Geometry: final body of the model. Coordinates: model frame, mm. A direction names the side the tool comes from. Coordinates: 2 decimals unless noted, no trailing zeros. Loops run counter-clockwise (first coordinate to the right, second up) from the corner with the lowest first, then second, coordinate; pieces in that order, holes last. Notation, with made-up numbers: M 60,-12 L 72,-12 A12 ccw 72,1 Z; hole C 80,78.5 d4. An arc over 180 degrees is marked long. Write item = value, one per line. Start each with the question number.
```python
from build123d import *

# Parameters (mm, degrees)
SKETCH1_W            = 25
SKETCH1_H            = 9.6
BOSS_EXTRUDE1_DEPTH  = 2
SKETCH3_R            = 2.3
CUT_EXTRUDE1_DEPTH   = 14.538463724
SKETCH4_W            = 20.2
SKETCH4_H            = 6.2
CUT_EXTRUDE2_DEPTH   = 0.27
SKETCH5_W            = 40
SKETCH5_H            = 20
BOSS_EXTRUDE2_DEPTH  = 4
M3_CLEARANCE_HOLE1_D = 3.2
SKETCH9_W            = 40
SKETCH9_H            = 2
BOSS_EXTRUDE4_DEPTH  = 20
BOSS_EXTRUDE5_DEPTH  = 1.5
FILLET1_R            = 2
FILLET1_OF_MIRROR1_R = 2
M3_CLEARANCE_HOLE2_D = 3.2


with BuildPart() as part:
    # Sketch1 → Boss-Extrude1 (new body)
    with BuildSketch(Plane(origin=(0, 0, 0), x_dir=(1, 0, 0), z_dir=(0, 1, 0))):
        Rectangle(SKETCH1_W, SKETCH1_H)
    extrude(amount=BOSS_EXTRUDE1_DEPTH)

    # Sketch3 → Cut-Extrude1 (cut, through all)
    with BuildSketch(Plane(origin=(0, 2, 0), x_dir=(1, 0, 0), z_dir=(0, 1, 0))):
        with Locations(Location((-7, 0, 0), (0, 0, 270))):
            Circle(SKETCH3_R)
        with Locations(Location((7, 0, 0), (0, 0, 270))):
            Circle(SKETCH3_R)
    extrude(amount=-CUT_EXTRUDE1_DEPTH, mode=Mode.SUBTRACT)

    # Sketch4 → Cut-Extrude2 (cut)
    with BuildSketch(Plane(origin=(0, 0, 0), x_dir=(1, 0, 0), z_dir=(0, 1, 0))):
        Rectangle(SKETCH4_W, SKETCH4_H)
    extrude(amount=CUT_EXTRUDE2_DEPTH, mode=Mode.SUBTRACT)

    # Sketch5 → Boss-Extrude2 (add)
    with BuildSketch(Plane(origin=(0, 2, 0), x_dir=(1, 0, 0), z_dir=(0, 1, 0))):
        Rectangle(SKETCH5_W, SKETCH5_H)
    extrude(amount=BOSS_EXTRUDE2_DEPTH)

    # M3 Clearance Hole1 (through all)
    with Locations(Plane(origin=(0, 2, 0), x_dir=(-1, 0, 0), z_dir=(0, -1, 0))):
        with Locations((-7, 0), (7, 0)):
            Hole(M3_CLEARANCE_HOLE1_D / 2)

    # Sketch9 → Boss-Extrude4 (add)
    with BuildSketch(Plane(origin=(0, 6, 0), x_dir=(1, 0, 0), z_dir=(0, 1, 0))):
        with Locations((0, 9)):
            Rectangle(SKETCH9_W, SKETCH9_H)
        with Locations((0, -9)):
            Rectangle(SKETCH9_W, SKETCH9_H)
    extrude(amount=BOSS_EXTRUDE4_DEPTH)

    # Sketch10 → Boss-Extrude5 (add)
    with BuildSketch(Plane.ZY.offset(12.5)):
        Polygon((-8, 6), (-8, 26), (0, 6), align=None)
        Polygon((8, 6), (0, 6), (8, 26), align=None)
    boss_extrude5 = extrude(amount=BOSS_EXTRUDE5_DEPTH)

    # Fillet1
    fillet1_edges = [part.edges().sort_by_distance(p)[0] for p in [
        (-13.25, 6, 0),
    ]]
    fillet(fillet1_edges, radius=FILLET1_R)

    # Mirror1: Boss-Extrude5 across plane
    add(boss_extrude5.mirror(Plane.ZY))

    # Fillet1 of Mirror1
    fillet1_of_mirror1_edges = [part.edges().sort_by_distance(p)[0] for p in [
        (13.25, 6, 0),
    ]]
    fillet(fillet1_of_mirror1_edges, radius=FILLET1_OF_MIRROR1_R)

    # M3 Clearance Hole2 (through all)
    with Locations(Plane.XY.offset(10)):
        with Locations((-17.5, 21), (17.5, 21), (17.5, 11), (-17.5, 11), (0, 21), (0, 11)):
            Hole(M3_CLEARANCE_HOLE2_D / 2)


solid = part.part
```
Item 1: Section query A-A (x = 17.5). Return the cut outline in (y, z).
Item 2: Pull-direction query (Y, two-part tool) for faces 1 (the cylindrical face through (-6.309, 1.147, 2.194)), 2 (the cylindrical face through (0.208, 22.586, -9.014)), 3 (the cylindrical face through (0.35, 9.44, -9.01)), 4 (the flat face through (0, 26, 9)); classes: released by +Y, released by -Y, zero draft, split by the parting line, or undercut.
Item 3: First-contact query: pin 1 (3 mm diameter, centred on x = -5, z = 0.5, fed in from -Y); pin 2 (1.9 mm diameter, centred on x = -17.5, y = 21, fed in from -Z) (1 decimal); pin 3 (3 mm diameter, centred on x = 18, z = -1.5, fed in from +Y); pin 4 (3.5 mm diameter, centred on x = 7, z = 0, fed in from -Y). Flat tips, straight axial feed; report the tip coordinate or a pass-through.
Item 4: Reachability of faces 5 (the flat face through (-14, 9, -2)), 6 (the flat face through (17, 16, -8)), 7 (the flat face through (0, 1, 4.8)), 8 (the flat face through (0, 0.27, 0)) from +Z, -Z, +X, -X, +Y, -Y: full face, straight path, thin tool, end or side. Return the list, or none.
Item 5: Section query B-B (z = 4). Return the cut outline in (x, y), plus the area to 3 significant figures.
Item 6: Section query C-C (x = 7). Return the cut outline in (y, z).
Item 7: Line query: line 1 (Y direction, x = -17.5, z = -8.55); line 2 (Z direction, x = 5, y = 20.25); line 3 (Y direction, x = -3, z = 8.75). Output: solid intervals per line, ascending. Write a range as from..to.
Item 8: Section query D-D (y = 5.5). Return the cut outline in (x, z).
Verdict:
q1.outline = M 2,-10 L 9.4,-10 L 9.4,-8 L 6,-8 L 6,8 L 9.4,8 L 9.4,10 L 2,10 Z; M 12.6,-10 L 19.4,-10 L 19.4,-8 L 12.6,-8 Z; M 12.6,8 L 19.4,8 L 19.4,10 L 12.6,10 Z; M 22.6,-10 L 26,-10 L 26,-8 L 22.6,-8 Z; M 22.6,8 L 26,8 L 26,10 L 22.6,10 Z
q2.face_1 = zero draft
q2.face_2 = undercut
q2.face_3 = undercut
q2.face_4 = released by +Y
q3.pin_1 = 0.27
q3.pin_2 = through
q3.pin_3 = 6
q3.pin_4 = 2
q4.face_5 = -X, +Y
q4.face_6 = +X, +Y
q4.face_7 = +Z, +X, -X, -Y
q4.face_8 = -Y
q5.outline = M -20,2 L -12.5,2 L -12.5,0 L 12.5,0 L 12.5,2 L 20,2 L 20,6 L 14,6 L 14,16 L 12.5,16 L 12.5,6 L -12.5,6 L -12.5,16 L -14,16 L -14,6 L -20,6 Z
q5.area = 240 mm2
q6.outline = M 0,-4.8 L 2,-4.8 L 2,-10 L 26,-10 L 26,-8 L 6,-8 L 6,-1.6 L 2,-1.6 L 2,-2.3 L 0.27,-2.3 L 0.27,-3.1 L 0,-3.1 Z; M 0,3.1 L 0.27,3.1 L 0.27,2.3 L 2,2.3 L 2,1.6 L 6,1.6 L 6,8 L 26,8 L 26,10 L 2,10 L 2,4.8 L 0,4.8 Z
q7.line_1 = 2..9.4, 12.6..19.4, 22.6..26
q7.line_2 = -10..-8, 8..10
q7.line_3 = 2..26
q8.outline = M -20,-10 L 20,-10 L 20,10 L -20,10 Z; hole C -7,0 d3.2; hole C 7,0 d3.2
